Geometry: see drawing. Coordinates: mm, zero at the bounding-box minimum. A direction names the side the tool comes from. Give positions to 0.01 mm unless a question says otherwise; leave off trailing zeros. Order: outer loops, then holes, each group sorted by start corner. A loop starts at its lowest first (then second) coordinate and runs counter-clockwise, first axis right, second up. Notation, with made-up numbers: (18.25, 62) - (36.25, 62) arc R5 cw to (36.25, 68) - close; hole circle Ø9 at (83.25, 81.25). An arc over 180 degrees is marked (long way). Write item = value, one per line. Start each with the question number.
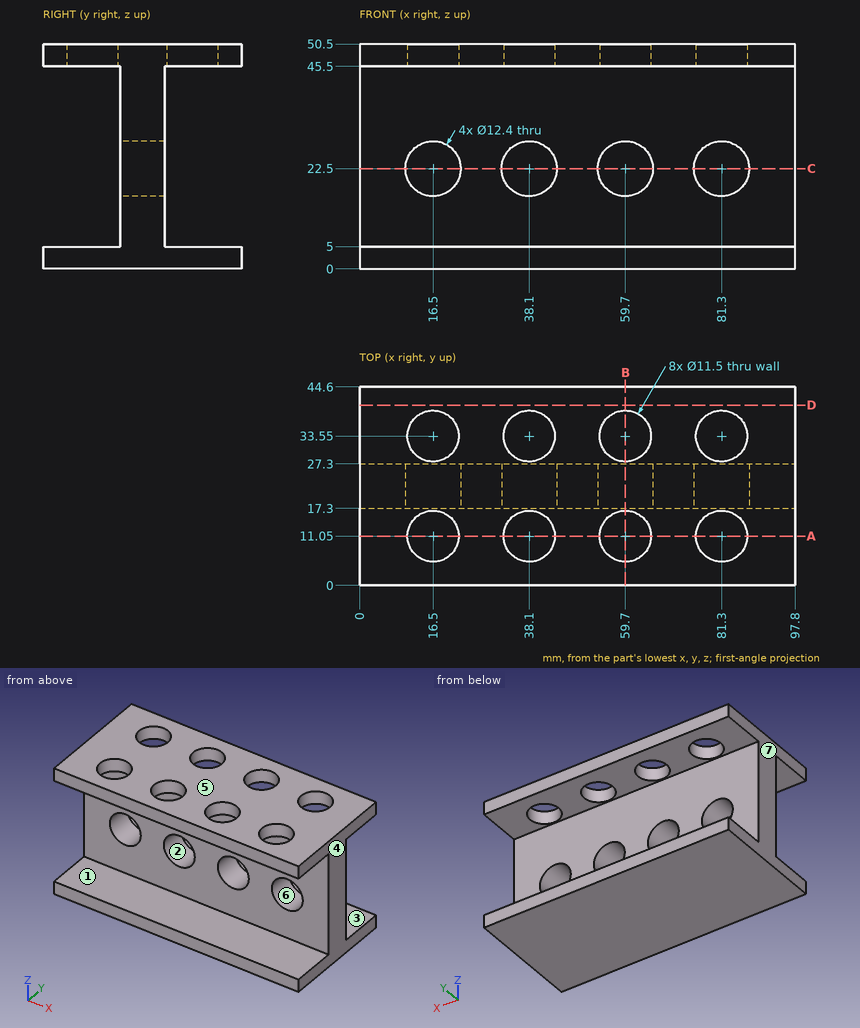
Q1. Pull-direction query (X, two-part tool) for the marked faces 4, 5, 6 and 7; classes: +X half, -X half, draft (parallel to the pull), parting line (faces both ways), or undercut.
Q2. Section C-C, the plane z = 22.5. Return the cut outline in (x, y), then the cut area to 3 significant figures.
Q3. Section A-A, the plane y = 11.05. Return the cut outline in (x, z), then the cut area to 3 significant figures.
Q4. Section D-D, the plane y = 40.5. Return the cut outline in (x, z), then the cut area to 3 significant figures.
Q5. Contact query for flat-ended pins moving along their axis: pin 1 (5 mm diameter, centred on x = 25, z = 40.5, fed in from -Y); pin 2 (16 mm diameter, centred on x = 38.1, z = 22.5, fed in from +Y); pin 3 (9 mm diameter, centred on x = 38.1, y = 11.05, fed in from +Z); pin 4 (10 mm diameter, centred on x = 81.3, z = 22.5, fed in from -Y). Output: stop coordinate, or through.
Q6. Set-up query: the marked faces 1, 2 and 3. Return all of +Z, -Z, +X, -X, +Y, -Y with unobstructed straight access to the full face (end or side cutting, diameter ignored); none if empty.
Q7. Material intervals for line 1 along Y through (x, z) = (81.3, 46.95); line 2 along X through (y, z) = (11, 47); line 3 along X through (y, z) = (20, 22), sorted ascending. Write a range as from..to.
Q8. Section B-B, the plane x = 59.7. Return the cut outline in (y, z).
The answers:
q1.face_4 = +X half
q1.face_5 = draft
q1.face_6 = undercut
q1.face_7 = -X half
q2.outline = (0, 17.3) - (10.3, 17.3) - (10.3, 27.3) - (0, 27.3) - close; (22.7, 17.3) - (31.9, 17.3) - (31.9, 27.3) - (22.7, 27.3) - close; (44.3, 17.3) - (53.5, 17.3) - (53.5, 27.3) - (44.3, 27.3) - close; (65.9, 17.3) - (75.1, 17.3) - (75.1, 27.3) - (65.9, 27.3) - close; (87.5, 17.3) - (97.8, 17.3) - (97.8, 27.3) - (87.5, 27.3) - close
q2.area = 482 mm²
q3.outline = (0, 0) - (97.8, 0) - (97.8, 5) - (0, 5) - close; (0, 45.5) - (10.75, 45.5) - (10.75, 50.5) - (0, 50.5) - close; (22.25, 45.5) - (32.35, 45.5) - (32.35, 50.5) - (22.25, 50.5) - close; (43.85, 45.5) - (53.95, 45.5) - (53.95, 50.5) - (43.85, 50.5) - close; (65.45, 45.5) - (75.55, 45.5) - (75.55, 50.5) - (65.45, 50.5) - close; (87.05, 45.5) - (97.8, 45.5) - (97.8, 50.5) - (87.05, 50.5) - close
q3.area = 748 mm²
q4.outline = (0, 0) - (97.8, 0) - (97.8, 5) - (0, 5) - close; (0, 45.5) - (97.8, 45.5) - (97.8, 50.5) - (0, 50.5) - close
q4.area = 978 mm²
q5.pin_1 = 17.3
q5.pin_2 = 27.3
q5.pin_3 = 5
q5.pin_4 = through
q6.face_1 = +X, -X, -Y
q6.face_2 = +Y, -Y
q6.face_3 = +X, -X, +Y
q7.line_1 = 0..5.3, 16.8..27.8, 39.3..44.6
q7.line_2 = 0..10.75, 22.25..32.35, 43.85..53.95, 65.45..75.55, 87.05..97.8
q7.line_3 = 0..10.32, 22.68..31.92, 44.28..53.52, 65.88..75.12, 87.48..97.8
q8.outline = (0, 0) - (44.6, 0) - (44.6, 5) - (27.3, 5) - (27.3, 16.3) - (17.3, 16.3) - (17.3, 5) - (0, 5) - close; (0, 45.5) - (5.3, 45.5) - (5.3, 50.5) - (0, 50.5) - close; (16.8, 45.5) - (17.3, 45.5) - (17.3, 28.7) - (27.3, 28.7) - (27.3, 45.5) - (27.8, 45.5) - (27.8, 50.5) - (16.8, 50.5) - close; (39.3, 45.5) - (44.6, 45.5) - (44.6, 50.5) - (39.3, 50.5) - close
